Autodesk Inventor part; units mm, degrees
ref_plane "작업 평면1" through (13.6, 4.8843, 7.5) normal (0, 0, -1) x (-1, 0, 0)
ref_plane "작업 평면2" through (13.6, 4.8843, 7.5) normal (0, 0, -1) x (-1, 0, 0)
ref_plane "작업 평면3" through (0, -1.8829, 13.6) normal (0, 0, -1) x (-1, 0, 0)
sketch "스케치1" plane through (0, 0, 0) normal (0, 0, 1) x (1, 0, 0)
  arc A0 (0, -7.65) -> (5.8602, 4.9173) centre (0, 0) ccw
  line L0 (0, -7.65) -> (0, -8.65)
  line L1 (0, -8.65) -> (13.6, -8.65)
  line L2 (13.6, -8.65) -> (13.6, 4.8843)
  line L3 (0, 0) -> (7.5, 0) construction
  line L4 (8.5089, 4.8843) -> (13.6, 4.8843)
  line L5 (0, 0) -> (0, 6.3672)
  line L6 (8.5089, 4.8843) -> (6.9333, 3.233)
  dimension "d0" = 15.3
  dimension "d1" = 1
  dimension "d2" = 13.6
revolve "회전1" add sketch "스케치1" angle 180 about axis through (0, 0, 0) along (0, -1, 0)
sketch "스케치3" plane through (0, 0, 0) normal (0, 0, 1) x (1, 0, 0)
  circle A0 centre (0, 0) radius 2
  dimension "d8" = 4
extrude "돌출2" cut sketch "스케치3" along normal mid plane 12
sketch "스케치4" plane through (0, 0, 0) normal (0, 0, 1) x (1, 0, 0)
  point P0 (0, 0)
  point P1 (0, 0)
sketch "스케치6" plane through (0, 0, 0) normal (0, 0, 1) x (1, 0, 0)
  point P0 (0, 0)
  point P1 (0, 0)
ref_plane "작업 평면1" through (13.6, 4.8843, 7.5) normal (0, 0, -1) x (-1, 0, 0)
ref_plane "작업 평면2" through (13.6, 4.8843, 7.5) normal (0, 0, -1) x (-1, 0, 0)
chamfer "모따기1" distance 2 angle 45 1 edges at (0, 4.8843, 13.6)
ref_plane "작업 평면3" through (0, -1.8829, 13.6) normal (0, 0, -1) x (-1, 0, 0)
ref_plane "작업 평면4" through (0, 0, 7.5) normal (0, 0, -1) x (-1, 0, 0)
fillet "모깎기2" radius 2 2 edges at (0, 2.8843, 13.6) (0, 4.8843, 11.6)
properties part number "ball socket"
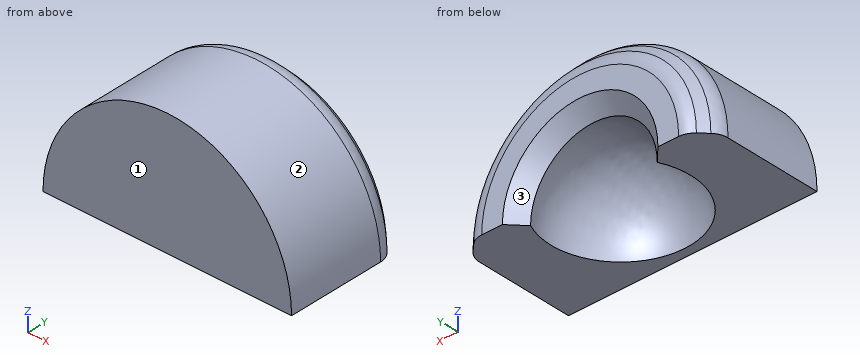
The model under review builds one solid part; all positions refer to its coordinate system, in mm. Face numbers are marked on the shaded views. Give positions to 0.01 mm unless a question says otherwise; leave off trailing zeros.
(1) For P1, Ø1, axis at y = -3.5, z = 5, coming from the +X side; P2, Ø4, axis at x = -7.5, y = 1.5, coming from the +Z side; P3, Ø5, axis at y = 2, z = 5, coming from the +X side, all flat-tipped, find the tip position at first contact; note any pin that passes through.
(2) To check wall thickness, follow L1, parallel to X at y = -6.25, z = 1.5; L2, parallel to X at y = -0.5, z = 1; L3, parallel to Z at x = -5.5, y = -0.25. State the ranges of each line that lie inside material, in increasing order.
(3) The part is to be moulded in two halves that separate along X. For the marked faces 1, 2 and 3, say which applies: released by +X, released by -X, zero draft, split by the parting line, or undercut.
Returned:
1. P1: stops at x = 12.83
1. P2: stops at z = 12.44
1. P3: stops at x = 13.37
2. L1: x = -13.52 to -4.15, 4.15 to 13.52
2. L2: x = -13.56 to -7.57, 7.57 to 13.56
2. L3: z = 5.31 to 12.44
3. face 1: zero draft
3. face 2: split by the parting line
3. face 3: undercut
